Geometry: see drawing. Coordinates: mm, zero at the bounding-box minimum. A direction names the side the tool comes from. Coordinates: 2 decimals unless noted, no trailing zeros. Order: outer loops, then holes, each group sorted by start corner. A loop starts at its lowest first (then second) coordinate and runs counter-clockwise, first axis right, second up. Notation, with made-up numbers: (61, 85) -> (115, 85) arc R25 cw to (115, 109) -> close; hole circle Ø2 at (58.5, 60.25). An arc over 180 degrees is marked (long way). Use one line per item in the form item = value.
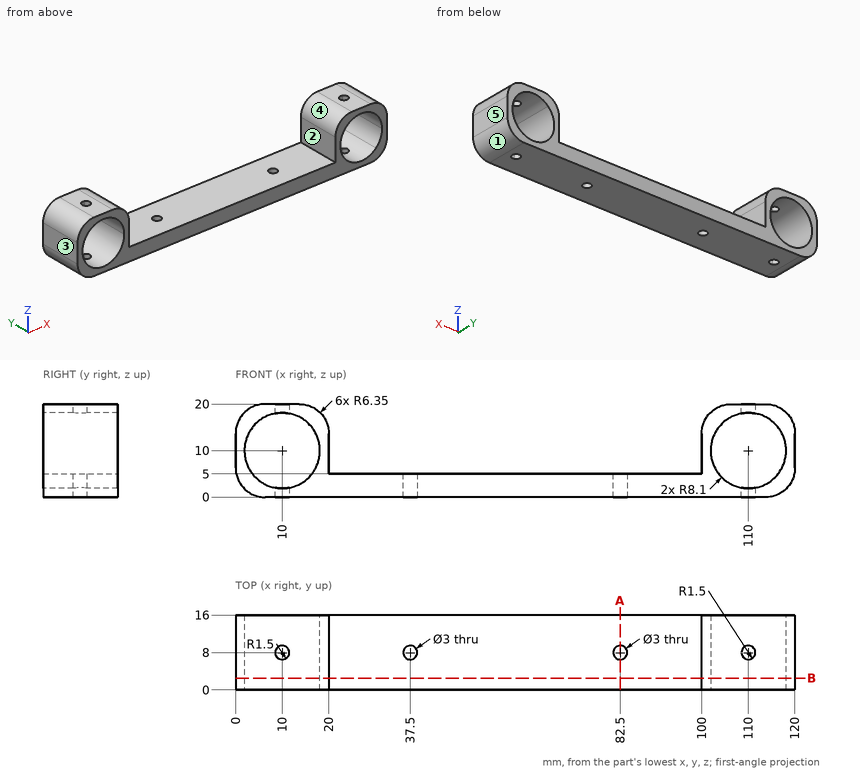
1) Pull-direction query (X, two-part tool) for the marked faces 1, 2 and 3; classes: released by +X, released by -X, zero draft, split by the parting line, or undercut.
Results found:
face_1 = released by +X
face_2 = undercut
face_3 = released by -X
2) Contact query for flat-ended pins moving along their axis: P1, Ø1, axis at y = 7, z = 3, coming from the +X side; P2, Ø1.5, axis at y = 3, z = 2.5, coming from the +X side. Output: stop coordinate, or through.
Results found:
P1 = 119.32
P2 = 119.19
3) Section A-A, the plane x = 82.5. Output: boundary loops of the cut face in (y, z).
Results found:
outline = (0, 0) -> (6.5, 0) -> (6.5, 5) -> (0, 5) -> close; (9.5, 0) -> (16, 0) -> (16, 5) -> (9.5, 5) -> close
4) Section B-B, the plane y = 2.5. Output: boundary loops of the cut face in (x, z).
Results found:
outline = (0, 6.35) arc R6.35 ccw to (6.35, 0) -> (113.65, 0) arc R6.35 ccw to (120, 6.35) -> (120, 13.65) arc R6.35 ccw to (113.65, 20) -> (106.35, 20) arc R6.35 ccw to (100, 13.65) -> (100, 5) -> (20, 5) -> (20, 13.65) arc R6.35 ccw to (13.65, 20) -> (6.35, 20) arc R6.35 ccw to (0, 13.65) -> close; hole circle Ø16.2 at (10, 10); hole circle Ø16.2 at (110, 10)
5) Access query for the marked faces 4 and 5. Directions: +Z, -Z, +X, -X, +Y, -Y. A direction counts if a zero-diameter tool reaches every point of the face in a straight line with its end or side. Return the directions, or none.
Results found:
face_4 = +Z, +Y, -Y
face_5 = +Z, -Z, +X, +Y, -Y
6) Material intervals for probe 1 along X at (y, z) = (7.75, 12.5); probe 2 along X at (y, z) = (12, 8.5); probe 3 along Y at (x, z) = (82.5, 2.45), sorted ascending. Write a range as from..to.
Results found:
probe_1 = 0..2.3, 17.7..20, 100..102.3, 117.7..120
probe_2 = 0..2.04, 17.96..20, 100..102.04, 117.96..120
probe_3 = 0..6.5, 9.5..16
